Check sheet for the modelled part. Datum: model origin and axes. Units: mm. Face numbers are marked on the shaded views. A direction names the side the tool comes from. Give positions to 0.01 mm unless a question says otherwise; leave off trailing zeros. Loops run counter-clockwise (first coordinate to the right, second up) from the corner with the lowest first, then second, coordinate; pieces in that order, holes last. Notation, with made-up numbers: (22, 14) -> (47, 14) arc R20 ccw to (47, 42) -> close; hole circle Ø7 at (85.5, -3.5). An arc over 180 degrees is marked (long way). Answer as CSV lines item,"result". Start each with the question number.
(1) Release check for a two-part mould opening along Y. For the marked faces 1, 2 and 3 record: pulls with the +Y half, pulls with the -Y half, needs draft (parallel to the pull), parting line crosses it, or undercut.
(2) Gauge pin test, flat ends, axial feed: pin 1 Ø1.5 at (y, z) = (6, 1.5) entering from +X; pin 2 Ø3 at (y, z) = (1, 8.5) entering from -X; pin 3 Ø2 at (x, y) = (6, 8) entering from +Z. Record the tip position at first contact, or that the pin passes through.
(3) Section check B-B on x = 0. Enter the section's corners in (y, z), plus the area to 3 significant figures.
(4) Access from +Z, -Z, +X, -X, +Y, -Y to the whole of each face (thin tool, end or side, straight path). Record for the marked faces 4, 5 and 6.
(5) Section check A-A on z = 11.5. Enter the section's corners in (x, y).
(6) Material ranges on line 1 (X direction, y = -1.75, z = 6.75); line 2 (Z direction, x = 1.5, y = 7.5); line 3 (X direction, y = 0.5, z = 8.5), recorded low to high. Write a range as from..to.
(7) Section check C-C on z = 1. Enter the section's corners in (x, y).
from build123d import *

# Parameters (mm, degrees)
F0_R     = 12.5
F1_DEPTH = 5
F2_R     = 4
F4_DEPTH = 10


with BuildPart() as f1:
    # F0 (on Top) → F1 (new body)
    with BuildSketch(Plane.XY):
        Circle(F0_R)
    extrude(amount=F1_DEPTH)

    # F2
    f2_edges = [f1.edges().sort_by_distance(p)[0] for p in [
        (-12.5, 0, 0),
    ]]
    fillet(f2_edges, radius=F2_R)

    # F3 (on face) → F4 (join)
    with BuildSketch(Plane.XY.offset(5)):
        with BuildLine():
            ThreePointArc((-1.8, 0), (-2.532233047, 1.767766953), (-4.3, 2.5))
            Line((-4.3, 2.5), (-4.3, -2.5))
            ThreePointArc((-4.3, -2.5), (-2.532233047, -1.767766953), (-1.8, 0))
        make_face()
        with BuildLine():
            ThreePointArc((-2.5, 6.6), (0, 4.1), (2.5, 6.6))
            Line((2.5, 6.6), (-2.5, 6.6))
        make_face()
        with BuildLine():
            Line((-2.5, -6.6), (2.5, -6.6))
            ThreePointArc((2.5, -6.6), (0, -4.1), (-2.5, -6.6))
        make_face()
        with BuildLine():
            Line((4.3, -2.5), (4.3, 2.5))
            ThreePointArc((4.3, 2.5), (1.8, 0), (4.3, -2.5))
        make_face()
    extrude(amount=F4_DEPTH)


solid = f1.part
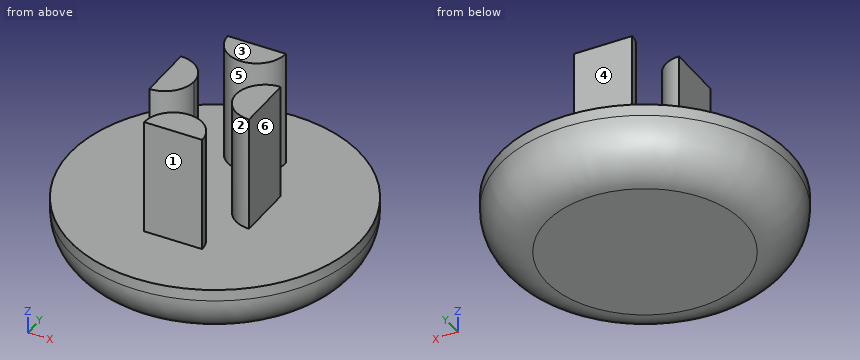
Working result:
1,face 1,"pulls with the -Y half"
1,face 2,"undercut"
1,face 3,"needs draft"
2,pin 1,"stops at x = 10.66"
2,pin 2,"stops at x = -4.3"
2,pin 3,"stops at z = 5"
3,outline,"(-12.5, 4) arc R4 ccw to (-8.5, 0) -> (8.5, 0) arc R4 ccw to (12.5, 4) -> (12.5, 5) -> (6.6, 5) -> (6.6, 15) -> (4.1, 15) -> (4.1, 5) -> (-4.1, 5) -> (-4.1, 15) -> (-6.6, 15) -> (-6.6, 5) -> (-12.5, 5) -> close"
3,area,"168 mm^2"
4,face 4,"+Z, +X, -X, +Y"
4,face 5,"+Z"
4,face 6,"+Z, +X, +Y, -Y"
5,outline,"(-4.3, -2.5) arc R2.5 ccw to (-4.3, 2.5) -> close; (-2.5, -6.6) -> (2.5, -6.6) arc R2.5 ccw to start; (-2.5, 6.6) arc R2.5 ccw to (2.5, 6.6) -> close; (4.3, -2.5) -> (4.3, 2.5) arc R2.5 ccw to start"
6,line 1,"x = -4.3..-2.51, 2.51..4.3"
6,line 2,"z = 0..5"
6,line 3,"x = -4.3..-1.85, 1.85..4.3"
7,outline,"circle Ø22.29 at (0, 0)"
